Verification items for the finished model (mm, model axes). Face numbers are marked on the shaded views. A direction names the side the tool comes from. Coordinates: 2 decimals unless noted, no trailing zeros. Write each loop counter-clockwise with the first axis right and the second up, starting at its lowest first coordinate (ties: lowest second). Pieces come first, ordered by that corner, then holes. Notation, with made-up numbers: (-39, -4) - (18, -4) arc R26 ccw to (18, 16) - close; hole circle Ø2 at (-36, 80). An arc over 180 degrees is marked (long way). Answer as CSV lines item,"result". Start each with the question number.
```python
from build123d import *

# Parameters (mm, degrees)
SKETCH3_W               = 48
SKETCH3_H               = 132
SKETCH3_W_2             = 24
SKETCH3_H_2             = 88
CUT_EXTRUDE1_DEPTH      = 7.5
CUT_EXTRUDE1_DEPTH_BACK = 7.5
SKETCH4_R               = 2.7
CUT_EXTRUDE2_DEPTH      = 6
SKETCH5_R               = 2.7
CUT_EXTRUDE3_DEPTH      = 6
SKETCH6_R               = 2.7
CUT_EXTRUDE4_DEPTH      = 6
SKETCH7_R               = 2.7
CUT_EXTRUDE5_DEPTH      = 6


with BuildPart() as part:
    # Sketch1 → Revolve1 (revolve)
    with BuildSketch(Plane.XY):
        with BuildLine():
            Line((0, 0), (0, 21.5))
            Line((0, 21.5), (0.5, 22))
            Line((0.5, 22), (4.5, 22))
            Line((4.5, 22), (5, 21.5))
            Line((5, 21.5), (5, 11.4))
            ThreePointArc((5, 11.4), (5.117157288, 11.117157288), (5.4, 11))
            Line((5.4, 11), (29.5, 11))
            Line((29.5, 11), (30, 10.5))
            Line((30, 10.5), (30, 0))
            Line((30, 0), (0, 0))
        make_face()
    revolve(axis=Axis((30, 0, 0), (-1, 0, 0)))

    # Sketch2 → Cut-Revolve1 (revolve, cut)
    with BuildSketch(Plane.XY):
        Polygon((0, 0), (0, 6), (1, 5), (29, 5), (30, 6), (30, 0), align=None)
    revolve(axis=Axis((30, 0, 0), (-1, 0, 0)), mode=Mode.SUBTRACT)

    # Sketch3 → Cut-Extrude1 (cut, two sides)
    with BuildSketch(Plane(origin=(0, 0, 0), x_dir=(0, 0, -1), z_dir=(1, 0, 0))) as cut_extrude1_sk:
        Rectangle(SKETCH3_W, SKETCH3_H)
        Rectangle(SKETCH3_W_2, SKETCH3_H_2, mode=Mode.SUBTRACT)
    extrude(amount=CUT_EXTRUDE1_DEPTH, mode=Mode.SUBTRACT)
    extrude(cut_extrude1_sk.sketch, amount=-CUT_EXTRUDE1_DEPTH_BACK, mode=Mode.SUBTRACT)

    # Sketch4 → Cut-Extrude2 (cut)
    with BuildSketch(Plane(origin=(-0.5, 0, 0), x_dir=(0, 0, -1), z_dir=(1, 0, 0))):
        with Locations((-7.75, 13.423393759)):
            Circle(SKETCH4_R)
    extrude(amount=CUT_EXTRUDE2_DEPTH, mode=Mode.SUBTRACT)

    # Sketch5 → Cut-Extrude3 (cut)
    with BuildSketch(Plane(origin=(-0.5, 0, 0), x_dir=(0, 0, -1), z_dir=(1, 0, 0))):
        with Locations((-7.75, -13.423393759)):
            Circle(SKETCH5_R)
    extrude(amount=CUT_EXTRUDE3_DEPTH, mode=Mode.SUBTRACT)

    # Sketch6 → Cut-Extrude4 (cut)
    with BuildSketch(Plane(origin=(-0.5, 0, 0), x_dir=(0, 0, -1), z_dir=(1, 0, 0))):
        with Locations((7.75, -13.423393759)):
            Circle(SKETCH6_R)
    extrude(amount=CUT_EXTRUDE4_DEPTH, mode=Mode.SUBTRACT)

    # Sketch7 → Cut-Extrude5 (cut)
    with BuildSketch(Plane(origin=(-0.5, 0, 0), x_dir=(0, 0, -1), z_dir=(1, 0, 0))):
        with Locations((7.75, 13.423393759)):
            Circle(SKETCH7_R)
    extrude(amount=CUT_EXTRUDE5_DEPTH, mode=Mode.SUBTRACT)


solid = part.part
```
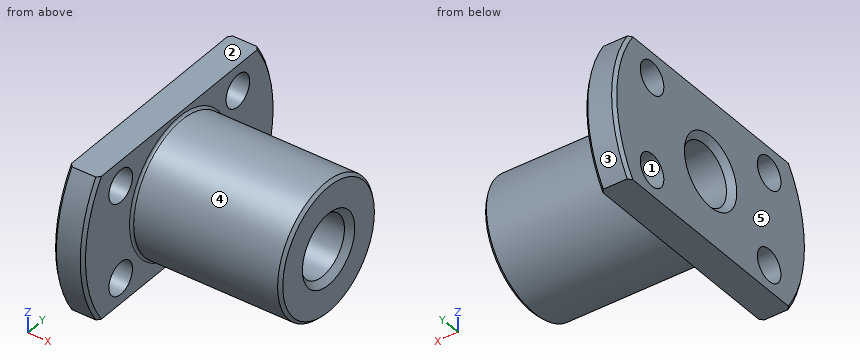
1. Depth check by flat-ended pin: P1, Ø7, axis at y = -13.42, z = 7.75, coming from the +X side; P2, Ø4, axis at x = 6, z = -4.5, coming from the +Y side; P3, Ø3, axis at x = 25, z = -6, coming from the +Y side; P4, Ø4.5, axis at y = -13.42, z = -7.75, coming from the -X side. Enter the tip coordinate at first touch or a pass-through.
2. Draft check along Z on the marked faces 1, 2 and 3. Enter one of: pulls with the +Z half, pulls with the -Z half, needs draft (parallel to the pull), parting line crosses it, or undercut.
3. Cross-section at A-A (z = 0). Record the cut outline in (x, y), and give its area (3 significant figures).
4. Cross-section at D-D (y = -14). Record the cut outline in (x, z).
5. Access from +Z, -Z, +X, -X, +Y, -Y to the whole of each face (thin tool, end or side, straight path). Record for the marked faces 4 and 5.
6. Cross-section at B-B (y = 0). Record the cut outline in (x, z), and give its area (3 significant figures).
7. Scan lines: line 1 along Y through (x, z) = (21, 0); line 2 along Y through (x, z) = (1.2, 7.75); line 3 along Z through (x, y) = (2.5, 15.5). Record each from-to range of solid material in increasing order. Write a range as from..to.
8. Cross-section at C-C (x = 2). Record the cut outline in (y, z), and give its area (3 significant figures).
Completed:
1,P1,"stops at x = 5"
1,P2,"stops at y = 21.77"
1,P3,"stops at y = 10.04"
1,P4,"passes through"
2,face 1,"undercut"
2,face 2,"pulls with the +Z half"
2,face 3,"parting line crosses it"
3,outline,"(0, -21.5) - (0.5, -22) - (4.5, -22) - (5, -21.5) - (5, -11.4) arc R0.4 cw to (5.4, -11) - (29.5, -11) - (30, -10.5) - (30, -6) - (29, -5) - (1, -5) - (0, -6) - close; (0, 6) - (1, 5) - (29, 5) - (30, 6) - (30, 10.5) - (29.5, 11) - (5.4, 11) arc R0.4 cw to (5, 11.4) - (5, 21.5) - (4.5, 22) - (0.5, 22) - (0, 21.5) - close"
3,area,"467 mm2"
4,outline,"(0, -12) - (5, -12) - (5, -10.39) - (0, -10.39) - close; (0, -5.11) - (5, -5.11) - (5, 5.11) - (0, 5.11) - close; (0, 10.39) - (5, 10.39) - (5, 12) - (0, 12) - close"
5,face 4,"+X"
5,face 5,"+Z, -Z, -X, +Y, -Y"
6,outline,"(0, -12) - (5, -12) - (5, -11.4) arc R0.4 cw to (5.4, -11) - (29.5, -11) - (30, -10.5) - (30, -6) - (29, -5) - (1, -5) - (0, -6) - close; (0, 6) - (1, 5) - (29, 5) - (30, 6) - (30, 10.5) - (29.5, 11) - (5.4, 11) arc R0.4 cw to (5, 11.4) - (5, 12) - (0, 12) - close"
6,area,"368 mm2"
7,line 1,"y = -11..-5, 5..11"
7,line 2,"y = -20.59..-16.12, -10.72..10.72, 16.12..20.59"
7,line 3,"z = -12..-9.48, -6.02..6.02, 9.48..12"
8,outline,"(-18.44, -12) - (18.44, -12) arc R22 ccw to (18.44, 12) - (-18.44, 12) arc R22 ccw to start; hole circle Ø5.4 at (-13.42, -7.75); hole circle Ø5.4 at (-13.42, 7.75); hole circle Ø10 at (0, 0); hole circle Ø5.4 at (13.42, -7.75); hole circle Ø5.4 at (13.42, 7.75)"
8,area,"831 mm2"
